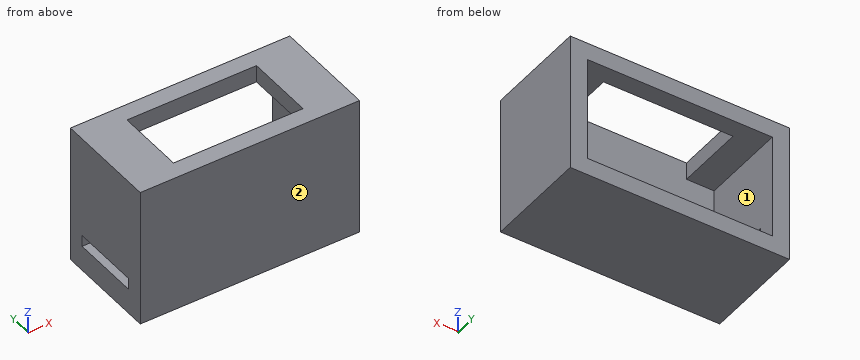
```python
from build123d import *

# Parameters (mm, degrees)
SKETCH1_W           = 38.1
SKETCH1_H           = 24.2
BOSS_EXTRUDE1_DEPTH = 18
SHELL1_T            = -3
SKETCH2_W           = 22.5
SKETCH2_H           = 12
CUT_EXTRUDE1_DEPTH  = 3
SKETCH3_W           = 2
SKETCH3_H           = 12
CUT_EXTRUDE2_DEPTH  = 3


with BuildPart() as part:
    # Sketch1 → Boss-Extrude1 (new body)
    with BuildSketch(Plane(origin=(0, 0, 0), x_dir=(1, 0, 0), z_dir=(0, 1, 0))):
        with Locations((-18.614066742, 14.699432105)):
            Rectangle(SKETCH1_W, SKETCH1_H)
    extrude(amount=BOSS_EXTRUDE1_DEPTH)

    # Shell1
    shell1_openings = [part.faces().sort_by_distance(p)[0] for p in [
        (-18.614066742, 18, -14.699432105),
    ]]
    offset(amount=SHELL1_T, openings=shell1_openings, kind=Kind.INTERSECTION)

    # Sketch2 → Cut-Extrude1 (cut)
    with BuildSketch(Plane.XY.offset(-2.599432105)):
        with Locations((-18.614066742, 9)):
            Rectangle(SKETCH2_W, SKETCH2_H)
    extrude(amount=-CUT_EXTRUDE1_DEPTH, mode=Mode.SUBTRACT)

    # Sketch3 → Cut-Extrude2 (cut)
    with BuildSketch(Plane.ZY.offset(37.664066742)):
        with Locations((-21.399432105, 9)):
            Rectangle(SKETCH3_W, SKETCH3_H)
    extrude(amount=-CUT_EXTRUDE2_DEPTH, mode=Mode.SUBTRACT)


solid = part.part
```
Geometry check sheet. Reference: the model listing, model coordinates, mm. Face numbers are marked on the shaded views. A direction names the side the tool comes from. Give positions to 0.01 mm unless a question says otherwise; leave off trailing zeros. Order: outer loops, then holes, each group sorted by start corner. A loop starts at its lowest first (then second) coordinate and runs counter-clockwise, first axis right, second up. Notation, with made-up numbers: (56, 62.25) - (71, 62.25) arc R11 cw to (71, 83.25) - close; hole circle Ø5 at (7.5, -22). An arc over 180 degrees is marked (long way). Write item = value, one per line. Start each with the question number.
1) Section check C-C (x = -14). Enter the section's corners in (y, z).
2) Scan lines: L1, parallel to Z at x = -11.5, y = 15.5; L2, parallel to Y at x = -9.5, z = -4; L3, parallel to X at y = 8.25, z = -4.75. Record each from-to range of solid material in increasing order.
3) Section check B-B (z = -21.5). Enter the section's corners in (x, y).
4) Access from +Z, -Z, +X, -X, +Y, -Y to the whole of each face (thin tool, end or side, straight path). Record for the marked faces 1 and 2.
5) Section check A-A (y = 9.5). Enter the section's corners in (x, z).
6) Section check D-D (x = -32.5). Enter the section's corners in (y, z), then the cut area to 3 significant figures.
Geometry check:
q1.outline = (0, -26.8) - (18, -26.8) - (18, -23.8) - (3, -23.8) - (3, -2.6) - (0, -2.6) - close; (15, -5.6) - (18, -5.6) - (18, -2.6) - (15, -2.6) - close
q2.L1 = -26.8 to -23.8, -5.6 to -2.6
q2.L2 = 0 to 3, 15 to 18
q2.L3 = -37.66 to -29.86, -7.36 to 0.44
q3.outline = (-37.66, 0) - (0.44, 0) - (0.44, 18) - (-2.56, 18) - (-2.56, 3) - (-37.66, 3) - close; (-37.66, 15) - (-34.66, 15) - (-34.66, 18) - (-37.66, 18) - close
q4.face_1 = +Y
q4.face_2 = +Z, -Z, +X, -X, -Y
q5.outline = (-37.66, -26.8) - (0.44, -26.8) - (0.44, -2.6) - (-7.36, -2.6) - (-7.36, -5.6) - (-2.56, -5.6) - (-2.56, -23.8) - (-34.66, -23.8) - (-34.66, -22.4) - (-37.66, -22.4) - close; (-37.66, -20.4) - (-34.66, -20.4) - (-34.66, -5.6) - (-29.86, -5.6) - (-29.86, -2.6) - (-37.66, -2.6) - close
q6.outline = (0, -26.8) - (18, -26.8) - (18, -23.8) - (3, -23.8) - (3, -5.6) - (18, -5.6) - (18, -2.6) - (0, -2.6) - close
q6.area = 163 mm2
